```python
from build123d import *

# Parameters (mm, degrees)
F0_R      = 25
F1_DEPTH  = 30
F2_R      = 1.5
F3_DEPTH  = 5
F4_R      = 6.35
F4_R_2    = 1.4224
F5_DEPTH  = 6.35
F6_DEPTH  = 9.525
F7_DEPTH  = 6.35
F8_DEPTH  = 9.525
F4_R_3    = 8
F9_DEPTH  = 20
F10_R     = 4
F11_DEPTH = 30.001
F4_R_4    = 10
F12_DEPTH = 2


with BuildPart() as f1:
    # F0 (on Top) → F1 (new body)
    with BuildSketch(Plane.XY):
        Circle(F0_R)
    extrude(amount=F1_DEPTH)

    # F2 (on face) → F3 (cut)
    with BuildSketch(Plane(origin=(0, 0, 0), x_dir=(1, 0, 0), z_dir=(0, 0, -1))):
        with Locations((0, 9.525)):
            Circle(F2_R)
        with Locations((-8.248891971, 4.7625)):
            Circle(F2_R)
        with Locations((-8.248891971, -4.7625)):
            Circle(F2_R)
        with Locations((0, -9.525)):
            Circle(F2_R)
        with Locations((8.248891971, -4.7625)):
            Circle(F2_R)
        with Locations((8.248891971, 4.7625)):
            Circle(F2_R)
    extrude(amount=-F3_DEPTH, mode=Mode.SUBTRACT)

    # F4 (on face) → F5 (cut)
    with BuildSketch(Plane.XY.offset(30)):
        with Locations((0, 16)):
            Circle(F4_R)
        with Locations((0, 16)):
            Circle(F4_R_2, mode=Mode.SUBTRACT)
    extrude(amount=-F5_DEPTH, mode=Mode.SUBTRACT)

    # F6 (cut): a face of the model
    f6_faces = [f1.faces().sort_by_distance(p)[0] for p in [
        (0, 16, 30),
    ]]
    extrude(f6_faces, amount=-F6_DEPTH, mode=Mode.SUBTRACT)

    # F4 (on face) → F7 (cut)
    with BuildSketch(Plane.XY.offset(30)):
        with Locations((0, -16)):
            Circle(F4_R)
        with Locations((0, -16)):
            Circle(F4_R_2, mode=Mode.SUBTRACT)
    extrude(amount=-F7_DEPTH, mode=Mode.SUBTRACT)

    # F4 (on face) → F8 (cut)
    with BuildSketch(Plane.XY.offset(30)):
        with Locations((0, -16)):
            Circle(F4_R_2)
    extrude(amount=-F8_DEPTH, mode=Mode.SUBTRACT)

    # F4 (on face) → F9 (cut)
    with BuildSketch(Plane.XY.offset(30)):
        with Locations((-13, 0)):
            Circle(F4_R_3)
    extrude(amount=-F9_DEPTH, mode=Mode.SUBTRACT)

    # F10 (on face) → F11 (cut, through all)
    with BuildSketch(Plane(origin=(0, 0, 0), x_dir=(1, 0, 0), z_dir=(0, 0, -1))):
        with Locations((-17, 0)):
            Circle(F10_R)
    extrude(amount=-F11_DEPTH, mode=Mode.SUBTRACT)

    # F4 (on face) → F12 (cut)
    with BuildSketch(Plane.XY.offset(30)):
        with Locations((-13, 0)):
            Circle(F4_R_4)
        with Locations((-13, 0)):
            Circle(F4_R_3, mode=Mode.SUBTRACT)
    extrude(amount=-F12_DEPTH, mode=Mode.SUBTRACT)


solid = f1.part
```
Read the model definition and answer for the solid it produces. Units are mm, in the model's axes. A direction names the side the tool comes from. Coordinates: 2 decimals unless noted, no trailing zeros. Loops run counter-clockwise (first coordinate to the right, second up) from the corner with the lowest first, then second, coordinate; pieces in that order, holes last. Notation, with made-up numbers: (-9, -5.75) - (13, -5.75) arc R25 cw to (13, 16.25) - close; hole circle Ø9 at (85, 45.5). An arc over 180 degrees is marked (long way). Answer in a Markdown table with one row per item.
1. Which of the six approach directions +Z, -Z, +X, -X, +Y, -Y give full straight-line access (tool end or side, diameter ignored) to faces 1 (the face through (-20.2, 2.4, 4.9)), 2 (the face through (0, 18, 23.65)), 3 (the face through (0, 10, 5))?
Conclusion:
| item | result |
|---|---|
| face 1 | +Z, -Z |
| face 2 | +Z |
| face 3 | -Z |
2. Given pin 1 (2.5 mm diameter, centred on x = -8.25, y = -4.76, fed in from -Z); pin 2 (1.5 mm diameter, centred on x = 15, z = 22, fed in from +Y); pin 3 (1.5 mm diameter, centred on y = -1, z = 10, fed in from -X), each flat-ended and moving along its own axis, determine where each tip first touches the part or whether it passes through.
Conclusion:
| item | result |
|---|---|
| pin 1 | stops at z = 5 |
| pin 2 | stops at y = 20.54 |
| pin 3 | stops at x = -25 |
3. Determine the mould class of faces 4 (the face through (5, 0, 30)), 5 (the face through (-9.4, -3.8, 2.5)), 6 (the face through (0, 16, 20.475)), 7 (the face through (23.846, 7.509, 14.79)) for opening direction X: +X half, -X half, draft (parallel to the pull), parting line (faces both ways), or undercut.
Conclusion:
| item | result |
|---|---|
| face 4 | draft |
| face 5 | undercut |
| face 6 | undercut |
| face 7 | parting line |
4. Find section A-A, the plane y = 2.5. Write down the section's boundary in (x, z).
Conclusion:
| item | result |
|---|---|
| outline | (-24.87, 0) - (-20.12, 0) - (-20.12, 10) - (-20.6, 10) - (-20.6, 28) - (-22.68, 28) - (-22.68, 30) - (-24.87, 30) - close; (-13.88, 0) - (24.87, 0) - (24.87, 30) - (-3.32, 30) - (-3.32, 28) - (-5.4, 28) - (-5.4, 10) - (-13.88, 10) - close |
5. Find section C-C, the plane x = -7.5. Write down the section's boundary in (y, z), then the cut area to 3 significant figures.
Conclusion:
| item | result |
|---|---|
| outline | (-23.85, 0) - (-6.06, 0) - (-6.06, 5) - (-3.46, 5) - (-3.46, 0) - (3.46, 0) - (3.46, 5) - (6.06, 5) - (6.06, 0) - (23.85, 0) - (23.85, 30) - (8.35, 30) - (8.35, 28) - (5.81, 28) - (5.81, 10) - (-5.81, 10) - (-5.81, 28) - (-8.35, 28) - (-8.35, 30) - (-23.85, 30) - close |
| area | 1,160 mm² |
6. Straight lines are drawn through the part: line 1 (Z direction, x = -22, y = -3); line 2 (Z direction, x = -12, y = -5); line 3 (X direction, y = 6, z = 19.25). For each, find the intervals that lie inside material, in ascending order.
Conclusion:
| item | result |
|---|---|
| line 1 | z = 0 to 28 |
| line 2 | z = 0 to 10 |
| line 3 | x = -24.27 to -18.29, -7.71 to 24.27 |
7. Find section D-D, the plane z = 7.5. Write down the section's boundary in (x, y), then the cut area to 3 significant figures.
Conclusion:
| item | result |
|---|---|
| outline | circle Ø50 at (0, 0); hole circle Ø8 at (-17, 0) |
| area | 1,910 mm² |
8. Find section B-B, the plane z = 3.75. Write down the section's boundary in (x, y) (1 decimal).
Conclusion:
| item | result |
|---|---|
| outline | circle Ø50 at (0, 0); hole circle Ø8 at (-17, 0); hole circle Ø3 at (-8.2, -4.8); hole circle Ø3 at (-8.2, 4.8); hole circle Ø3 at (0, -9.5); hole circle Ø3 at (0, 9.5); hole circle Ø3 at (8.2, -4.8); hole circle Ø3 at (8.2, 4.8) |
